```python
from build123d import *

# Parameters (mm, degrees)
SKETCH_1_R      = 2.5
EXTRUDE_1_DEPTH = 3


with BuildPart() as part:
    # 스케치1 → 보스-돌출1 (new body)
    with BuildSketch(Plane.XY):
        with BuildLine():
            Line((6.706268494, 10.103683016), (6.037882178, 5.957406269))
            Line((6.037882178, 5.957406269), (-1.376355668, 5.957406269))
            Line((-1.376355668, 5.957406269), (-3.724392512, 3.336000662))
            ThreePointArc((-3.724392512, 3.336000662), (-4.67022283, 1.785782383), (-5, 0))
            Line((-5, 0), (-5, -11.820871263))
            Line((-5, -11.820871263), (-3.253479839, -11.820871263))
            Line((-3.253479839, -11.820871263), (1.87605446, -7.031414053))
            Line((1.87605446, -7.031414053), (1.87605446, -4.634697365))
            ThreePointArc((1.87605446, -4.634697365), (2.980195691, -4.014776911), (3.893195608, -3.13736003))
            Line((3.893195608, -3.13736003), (9.172978659, -3.13736003))
            Line((9.172978659, -3.13736003), (14.557074242, 2.286312605))
            Line((14.557074242, 2.286312605), (14.557074242, 5.198022376))
            Line((14.557074242, 5.198022376), (9.615353398, 10.103683016))
            Line((9.615353398, 10.103683016), (6.706268494, 10.103683016))
        make_face()
        Circle(SKETCH_1_R, mode=Mode.SUBTRACT)
    extrude(amount=EXTRUDE_1_DEPTH)


solid = part.part
```
Can you work these out from the model? Positions are in its coordinate system, mm. A direction names the side the tool comes from. Give positions to 0.01 mm unless a question says otherwise; leave off trailing zeros. Order: outer loops, then holes, each group sorted by start corner. A loop starts at its lowest first (then second) coordinate and runs counter-clockwise, first axis right, second up. Notation, with made-up numbers: (63.25, -15.5) - (119.25, -15.5) arc R20 ccw to (119.25, -2.5) - close; hole circle Ø10 at (80.5, 56). An arc over 180 degrees is marked (long way). Use a Markdown table: item, result. Add a question column.
Q1. If we section it at A-A on z = 2.1: Write out the boundary of the cut face in (x, y).
Q2. If we section it at B-B on x = 0: Write out the boundary of the cut face in (y, z).
Q3. If we section it at D-D on x = 13: Write out the boundary of the cut face in (y, z).
Q4. On a 3-axis mill with a long thin cutter (end or side, diameter ignored), from which of +Z, -Z, +X, -X, +Y, -Y can I reach the whole of each face in a straight line? I mean faces 4 (the flat face through (1.876, -6, 1)), 5 (the flat face through (-5, -6, 1)). Say none if no direction works.
Q5. If we section it at C-C on y = -1.5: Write out the boundary of the cut face in (x, z).
Q6. If we mould it in two halves opening along Y, with no side actions, what happens to faces 1 (the flat face through (2, 5.957, 1)), 2 (the flat face through (11.83, -0.46, 1.48)), 3 (the cylindrical face through (-0.54, -2.44, 1.48))? For each: released by +Y, released by -Y, zero draft, split by the parting line, or undercut.
Q7. I'm going to push flat-ended pins straight in: pin 1 (1 mm diameter, centred on y = -2.5, z = 1, fed in from +X); pin 2 (1.5 mm diameter, centred on x = 8, z = 2.5, fed in from -Y); pin 3 (4.5 mm diameter, centred on x = 0, y = 0, fed in from +Z); pin 4 (1.5 mm diameter, centred on x = 2, z = 1.5, fed in from +Y). Where does each tip first touch, or does it pass through?
Q8. Please list where these lines run through material, in increasing order: line 1 along X through (y, z) = (-6.25, 1.05); line 2 along Y through (x, z) = (0, 2.1); line 3 along Y through (x, z) = (8, 1.65).
Answers follow:
| question | item | result |
|---|---|---|
| 1 | outline | (-5, -11.82) - (-3.25, -11.82) - (1.88, -7.03) - (1.88, -4.63) arc R5 ccw to (3.89, -3.14) - (9.17, -3.14) - (14.56, 2.29) - (14.56, 5.2) - (9.62, 10.1) - (6.71, 10.1) - (6.04, 5.96) - (-1.38, 5.96) - (-3.72, 3.34) arc R5 ccw to (-5, 0) - close; hole circle Ø5 at (0, 0) |
| 2 | outline | (-8.78, 0) - (-2.5, 0) - (-2.5, 3) - (-8.78, 3) - close; (2.5, 0) - (5.96, 0) - (5.96, 3) - (2.5, 3) - close |
| 3 | outline | (0.72, 0) - (6.74, 0) - (6.74, 3) - (0.72, 3) - close |
| 4 | face 4 | +Z, -Z, +X, -Y |
| 4 | face 5 | +Z, -Z, -X, +Y, -Y |
| 5 | outline | (-5, 0) - (-2, 0) - (-2, 3) - (-5, 3) - close; (2, 0) - (10.8, 0) - (10.8, 3) - (2, 3) - close |
| 6 | face 1 | released by +Y |
| 6 | face 2 | released by -Y |
| 6 | face 3 | undercut |
| 7 | pin 1 | stops at x = 10.3 |
| 7 | pin 2 | stops at y = -3.14 |
| 7 | pin 3 | passes through |
| 7 | pin 4 | stops at y = 5.96 |
| 8 | line 1 | x = -5 to 1.88 |
| 8 | line 2 | y = -8.78 to -2.5, 2.5 to 5.96 |
| 8 | line 3 | y = -3.14 to 10.1 |
